```python
from build123d import *

# Parameters (mm, degrees)
SKETCH1_R           = 20
BOSS_EXTRUDE1_DEPTH = 200
FILLET2_R           = 15
BOSS_EXTRUDE2_START = -200
SKETCH2_W           = 2
SKETCH2_H           = 10
BOSS_EXTRUDE2_DEPTH = 20
SKETCH3_R           = 2.5
CUT_EXTRUDE1_DEPTH  = 11


with BuildPart() as part:
    # Sketch1 → Boss-Extrude1 (new, symmetric)
    with BuildSketch(Plane.XY):
        Circle(SKETCH1_R)
    extrude(amount=BOSS_EXTRUDE1_DEPTH, both=True)

    # Fillet2
    fillet2_edges = [part.edges().sort_by_distance(p)[0] for p in [
        (-20, 0, 200),
    ]]
    fillet(fillet2_edges, radius=FILLET2_R)

    # Sketch2 → Boss-Extrude2 (add)
    with BuildSketch(Plane.XY.offset(BOSS_EXTRUDE2_START)):
        with Locations((-9, 0)):
            Rectangle(SKETCH2_W, SKETCH2_H)
        with Locations((9, 0)):
            Rectangle(SKETCH2_W, SKETCH2_H)
    extrude(amount=-BOSS_EXTRUDE2_DEPTH)

    # Sketch3 → Cut-Extrude1 (cut, symmetric)
    with BuildSketch(Plane(origin=(0, 0, 0), x_dir=(0, 0, -1), z_dir=(1, 0, 0))):
        with Locations((215, 0)):
            Circle(SKETCH3_R)
    extrude(amount=CUT_EXTRUDE1_DEPTH, both=True, mode=Mode.SUBTRACT)


solid = part.part
```
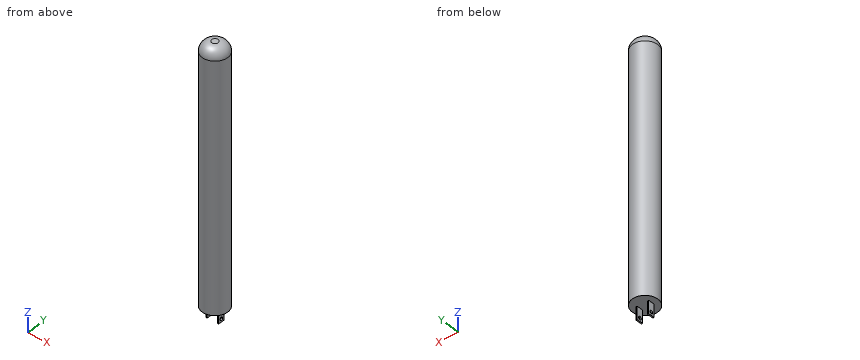
Work out the finished part from the listing and answer in its coordinate system (mm). Give positions to 0.01 mm unless a question says otherwise; leave off trailing zeros. Order: outer loops, then holes, each group sorted by start corner. A loop starts at its lowest first (then second) coordinate and runs counter-clockwise, first axis right, second up. Notation, with made-up numbers: (36, 57.5) -> (41, 57.5) arc R30 ccw to (41, 80.5) -> close; hole circle Ø9 at (74.5, 37.5). An arc over 180 degrees is marked (long way). Answer as CSV lines item,"result". Start each with the question number.
(1) Consider line 1 along Y through (x, z) = (9, -215); line 2 along X through (y, z) = (1, -190.5); line 3 along Y through (x, z) = (1.5, -136). Determine where each line is inside the solid, lowest interval first.
(2) Each of these flat-tipped pins is pushed along its axis until it touches: pin 1 Ø8 at (y, z) = (-13, -118) entering from +X; pin 2 Ø4 at (y, z) = (8.5, 156.5) entering from +X; pin 3 Ø2 at (x, y) = (-6, -14) entering from -Z. Where does it stop, or does it pass through?
(3) Section A-A, the plane z = -130 is taken. Write down the section's boundary in (x, y), plus the area to 3 significant figures.
Entries:
1,line 1,"-5 to -2.5, 2.5 to 5"
1,line 2,"-19.97 to 19.97"
1,line 3,"-19.94 to 19.94"
2,pin 1,"x = 17.86"
2,pin 2,"x = 18.91"
2,pin 3,"z = -200"
3,outline,"circle Ø40 at (0, 0)"
3,area,"1,260 mm²"
